Can you work these out from the model? Positions are in its coordinate system, mm. Face numbers are marked on the shaded views. A direction names the side the tool comes from. Give positions to 0.01 mm unless a question says otherwise; leave off trailing zeros. Loops run counter-clockwise (first coordinate to the right, second up) from the corner with the lowest first, then second, coordinate; pieces in that order, holes last. Notation, with made-up numbers: (-15.5, 32) - (34.5, 32) arc R20 ccw to (34.5, 54) - close; hole circle Ø11 at (61, -34.75). An arc over 180 degrees is marked (long way). Answer as a JSON object with one key per item and string values.
```python
from build123d import *

# Parameters (mm, degrees)
BOSS_EXTRUDE1_DEPTH = 75
CUT_EXTRUDE1_DEPTH  = 2.25
SKETCH3_W           = 11.7
SKETCH3_H           = 2.25
BOSS_EXTRUDE2_DEPTH = 15
SKETCH4_W           = 11.7
SKETCH4_H           = 5.5
BOSS_EXTRUDE3_DEPTH = 7.5
SKETCH5_W           = 11.7
SKETCH5_H           = 2
BOSS_EXTRUDE4_DEPTH = 15
SKETCH6_R           = 5
CUT_EXTRUDE2_DEPTH  = 2.25
CHAMFER1_SIZE       = 10
CHAMFER2_SIZE       = 10


with BuildPart() as part:
    # Sketch1 → Boss-Extrude1 (new body)
    with BuildSketch(Plane.XY):
        Polygon((-15, 0), (15, 0), (15, -2.25), (10.1, -2.25), (10.1, -4.41), (13.85, -4.41), (13.85, -5.88), (5.85, -5.88), (5.85, -2.25), (-5.85, -2.25), (-5.85, -5.88), (-13.85, -5.88), (-13.85, -4.41), (-10.1, -4.41), (-10.1, -2.25), (-15, -2.25), align=None)
    extrude(amount=BOSS_EXTRUDE1_DEPTH)

    # Sketch2 → Cut-Extrude1 (cut)
    with BuildSketch(Plane(origin=(0, 0, 0), x_dir=(1, 0, 0), z_dir=(0, 1, 0))):
        with BuildLine():
            Line((2.5, -11), (2.5, 0))
            Line((2.5, 0), (-2.5, 0))
            Line((-2.5, 0), (-2.5, -11))
            ThreePointArc((-2.5, -11), (0, -13.5), (2.5, -11))
        make_face()
    extrude(amount=-CUT_EXTRUDE1_DEPTH, mode=Mode.SUBTRACT)

    # Sketch3 → Boss-Extrude2 (add)
    with BuildSketch(Plane.XY.offset(75)):
        with Locations((0, -1.125)):
            Rectangle(SKETCH3_W, SKETCH3_H)
    extrude(amount=BOSS_EXTRUDE2_DEPTH)

    # Sketch4 → Boss-Extrude3 (add)
    with BuildSketch(Plane(origin=(0, 0, 0), x_dir=(1, 0, 0), z_dir=(0, 1, 0))):
        with Locations((0, -87.25)):
            Rectangle(SKETCH4_W, SKETCH4_H)
    extrude(amount=BOSS_EXTRUDE3_DEPTH)

    # Sketch5 → Boss-Extrude4 (add)
    with BuildSketch(Plane(origin=(0, 0, 84.5), x_dir=(-1, 0, 0), z_dir=(0, 0, -1))):
        with Locations((0, 1)):
            Rectangle(SKETCH5_W, SKETCH5_H)
    extrude(amount=BOSS_EXTRUDE4_DEPTH)

    # Sketch6 → Cut-Extrude2 (cut)
    with BuildSketch(Plane(origin=(0, 0, 0), x_dir=(1, 0, 0), z_dir=(0, 1, 0))):
        with Locations((0, -17)):
            Circle(SKETCH6_R)
    extrude(amount=-CUT_EXTRUDE2_DEPTH, mode=Mode.SUBTRACT)

    # Chamfer1
    chamfer1_edges = [part.edges().sort_by_distance(p)[0] for p in [
        (15, -1.125, 0),
    ]]
    chamfer(chamfer1_edges, length=CHAMFER1_SIZE)

    # Chamfer2
    chamfer2_edges = [part.edges().sort_by_distance(p)[0] for p in [
        (-15, -1.125, 0),
    ]]
    chamfer(chamfer2_edges, length=CHAMFER2_SIZE)


solid = part.part
```
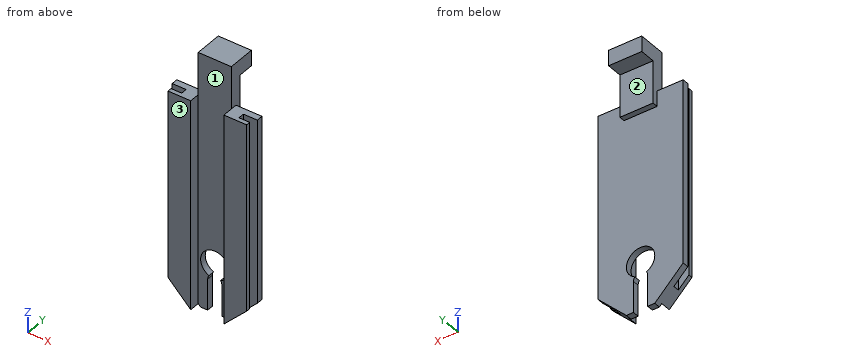
1) Imagine slicing it at D-D on z = 38. Write out the boundary of the cut face in (x, y), and give its area (3 significant figures).
Check sheet entries:
{"outline": "(-15, -2.25) - (-10.1, -2.25) - (-10.1, -4.41) - (-13.85, -4.41) - (-13.85, -5.88) - (-5.85, -5.88) - (-5.85, -2.25) - (5.85, -2.25) - (5.85, -5.88) - (13.85, -5.88) - (13.85, -4.41) - (10.1, -4.41) - (10.1, -2.25) - (15, -2.25) - (15, 0) - (-15, 0) - close", "area": "109 mm2"}
2) I need wall thicknesses on L1, parallel to Y at x = -10.5, z = 7; L2, parallel to X at y = -3.75, z = 60.5; L3, parallel to X at y = -0.8, z = 17. Which ranges of each line are inside material? Lowest first, please.
Check sheet entries:
{"L1": "-5.88 to -4.41, -2.25 to 0", "L2": "-10.1 to -5.85, 5.85 to 10.1", "L3": "-15 to -5, 5 to 15"}
3) Imagine slicing it at B-B on z = 17. Write out the boundary of the cut face in (x, y).
Check sheet entries:
{"outline": "(-15, -2.25) - (-10.1, -2.25) - (-10.1, -4.41) - (-13.85, -4.41) - (-13.85, -5.88) - (-5.85, -5.88) - (-5.85, -2.25) - (-5, -2.25) - (-5, 0) - (-15, 0) - close; (5, -2.25) - (5.85, -2.25) - (5.85, -5.88) - (13.85, -5.88) - (13.85, -4.41) - (10.1, -4.41) - (10.1, -2.25) - (15, -2.25) - (15, 0) - (5, 0) - close"}
4) I'm going to push flat-ended pins straight in: P1, Ø8, axis at x = -9.5, z = 39, coming from the +Y side; P2, Ø2.5, axis at y = -1.5, z = 3.5, coming from the +X side; P3, Ø1.1, axis at y = -4, z = 34.5, coming from the -X side; P4, Ø3, axis at y = 5, z = 79.5, coming from the +X side. Where does each tip first touch, or does it pass through?
Check sheet entries:
{"P1": "y = 0", "P2": "x = 9.75", "P3": "x = -13.85", "P4": "through"}
5) Imagine slicing it at A-A on x = -11.5. Write out the boundary of the cut face in (y, z).
Check sheet entries:
{"outline": "(-5.88, 6.5) - (-4.41, 6.5) - (-4.41, 75) - (-5.88, 75) - close; (-2.25, 6.5) - (0, 6.5) - (0, 75) - (-2.25, 75) - close"}
6) Which directions (+Z, -Z, +X, -X, +Y, -Y) give clear straight access to the entire face, cutting with the end or side of a thin tool? Please do the marked faces 1, 2 and 3.
Check sheet entries:
{"face 1": "+Z, -Z, -Y", "face 2": "-Z, +X, -X, +Y", "face 3": "+Z, -Z, +X, -X, -Y"}
7) Imagine slicing it at C-C on x = 0. Write out the boundary of the cut face in (y, z), and give its area (3 significant figures).
Check sheet entries:
{"outline": "(-2.25, 22) - (0, 22) - (0, 69.5) - (2, 69.5) - (2, 84.5) - (7.5, 84.5) - (7.5, 90) - (-2.25, 90) - close", "area": "224 mm2"}
